CAD build for the part. Positions are in the model's coordinates, mm. Face numbers are marked on the shaded views. A direction names the side the tool comes from. Give positions to 0.01 mm unless a question says otherwise; leave off trailing zeros. Write each loop counter-clockwise with the first axis right and the second up, starting at its lowest first coordinate (ties: lowest second). Pieces come first, ordered by that corner, then holes. Notation, with made-up numbers: M -18,31 L 18,31 A24 cw 18,51 Z; hole C -3.5,61 d9. An arc over 180 degrees is marked long. One line per question, with ' | ' between items. Start each with the question number.
1. Cut at B-B, the plane z = 0.75. Write the cut outline in (x, y), then the cut area to 3 significant figures.
2. Pull direction Z, two halves, no side cores. Call the marked faces 4, 5, 6 and 7: released by +Z, released by -Z, zero draft, split by the parting line, or undercut.
3. Which spindle directions (+Z, -Z, +X, -X, +Y, -Y) get a long thin tool onto all of the face, cutting with end or side? Do the marked faces 1, 2 and 3. Say none if no direction does.
4. Cut at C-C, the plane x = 5.5. Write the cut outline in (y, z).
5. Wall check: L1, parallel to Z at x = -2.5, y = 14.5; L2, parallel to X at y = 41, z = 3.5; L3, parallel to X at y = 6.5, z = -1.75. Give the ranges that are in metal, low to high.
6. Cut at D-D, the plane y = 13.5. Write the cut outline in (x, z).
7. Flat gauge pins, fed straight in: pin 1 (3.5 mm diameter, centred on y = 42.5, z = 0.5, fed in from +X); pin 2 (4 mm diameter, centred on x = 0.5, z = -3.5, fed in from +Y); pin 3 (5.5 mm diameter, centred on y = 46, z = 3.5, fed in from -X); pin 4 (1.6 mm diameter, centred on x = 23, z = 3.5, fed in from +Y). Where does each tip first touch, or does it go through?
8. Cut at A-A, the plane y = 46. Write the cut outline in (x, z).
```python
from build123d import *

# Parameters (mm, degrees)
SKETCH1_W          = 49
SKETCH1_H          = 17
SKETCH1_W_2        = 41
SKETCH1_H_2        = 13
EXTRUDE1_DEPTH     = 50
CUT_EXTRUDE3_DEPTH = 21
SKETCH3_W          = 49
SKETCH3_H          = 17
EXTRUDE2_DEPTH     = 2
FILLET1_R          = 2


with BuildPart() as part:
    # Sketch1 → Extrude1 (new body)
    with BuildSketch(Plane(origin=(0, 0, 0), x_dir=(1, 0, 0), z_dir=(0, 1, 0))):
        Rectangle(SKETCH1_W, SKETCH1_H)
        Rectangle(SKETCH1_W_2, SKETCH1_H_2, mode=Mode.SUBTRACT)
    extrude(amount=EXTRUDE1_DEPTH)

    # Sketch2 → Cut-Extrude3 (cut)
    with BuildSketch(Plane.XY.offset(8.5)):
        with BuildLine():
            Line((-21.439339828, 37.560660172), (-22.5, 38.621320344))
            Line((-22.5, 38.621320344), (-22.5, 50))
            Line((-22.5, 50), (-24.5, 50))
            Line((-24.5, 50), (-24.5, 35))
            Line((-24.5, 35), (-22.5, 35))
            ThreePointArc((-22.5, 35), (-21.114180701, 35.925974851), (-21.439339828, 37.560660172))
        make_face()
        with BuildLine():
            Line((24.5, 50), (22.5, 50))
            Line((22.5, 50), (22.5, 38.621320344))
            Line((22.5, 38.621320344), (21.439339828, 37.560660172))
            ThreePointArc((21.439339828, 37.560660172), (21.114180701, 35.925974851), (22.5, 35))
            Line((22.5, 35), (24.5, 35))
            Line((24.5, 35), (24.5, 50))
        make_face()
    extrude(amount=-CUT_EXTRUDE3_DEPTH, mode=Mode.SUBTRACT)

    # Sketch3 → Extrude2 (add)
    with BuildSketch(Plane.XZ):
        Rectangle(SKETCH3_W, SKETCH3_H)
    extrude(amount=EXTRUDE2_DEPTH)

    # Fillet1
    fillet1_edges = [part.edges().sort_by_distance(p)[0] for p in [
        (-24.5, 16.5, -8.5),
        (-24.5, 16.5, 8.5),
        (24.5, 16.5, -8.5),
        (24.5, 16.5, 8.5),
        (-24.5, -2, 0),
        (0, -2, -8.5),
        (24.5, -2, 0),
        (0, -2, 8.5),
    ]]
    fillet(fillet1_edges, radius=FILLET1_R)


solid = part.part
```
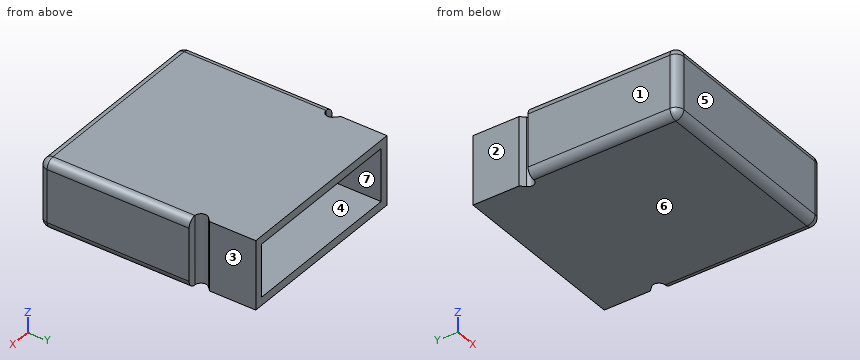
Here are the results:
1) outline: M -24.5,0 A2 ccw -22.5,-2 L 22.5,-2 A2 ccw 24.5,0 L 24.5,35 L 22.5,35 A1.5 cw 21.44,37.56 L 22.5,38.62 L 22.5,50 L 20.5,50 L 20.5,0 L -20.5,0 L -20.5,50 L -22.5,50 L -22.5,38.62 L -21.44,37.56 A1.5 cw -22.5,35 L -24.5,35 Z | area: 429 mm^2
2) face 4: undercut | face 5: zero draft | face 6: released by -Z | face 7: undercut
3) face 1: +Z, -Z, -X, +Y, -Y | face 2: +Z, -Z, -X, +Y | face 3: +Z, -Z, +X, +Y
4) outline: M -2,-6.5 A2 ccw 0,-8.5 L 50,-8.5 L 50,-6.5 L 0,-6.5 L 0,6.5 L 50,6.5 L 50,8.5 L 0,8.5 A2 ccw -2,6.5 Z
5) L1: -8.5 to -6.5, 6.5 to 8.5 | L2: -22.5 to -20.5, 20.5 to 22.5 | L3: -24.5 to -20.5, 20.5 to 24.5
6) outline: M -24.5,-6.5 A2 ccw -22.5,-8.5 L 22.5,-8.5 A2 ccw 24.5,-6.5 L 24.5,6.5 A2 ccw 22.5,8.5 L -22.5,8.5 A2 ccw -24.5,6.5 Z; hole M -20.5,-6.5 L 20.5,-6.5 L 20.5,6.5 L -20.5,6.5 Z
7) pin 1: x = 22.5 | pin 2: y = 0 | pin 3: x = -22.5 | pin 4: y = 50
8) outline: M -22.5,-8.5 L 22.5,-8.5 L 22.5,8.5 L -22.5,8.5 Z; hole M -20.5,-6.5 L 20.5,-6.5 L 20.5,6.5 L -20.5,6.5 Z
